Can you work these out from the model? Positions are in its coordinate system, mm. A direction names the side the tool comes from. Round coordinates to 2 decimals unless told otherwise and drop trailing zeros. Loops run counter-clockwise (first coordinate to the right, second up) from the corner with the lowest first, then second, coordinate; pieces in that order, holes last. Notation, with made-up numbers: M 14,8 L 44,8 A29 cw 44,47 Z; hole C 32.25,-32.5 d7. An arc over 180 degrees is marked long. Answer as CSV lines item,"result".
from build123d import *

# Parameters (mm, degrees)
SKETCH1_W           = 55.54
SKETCH1_H           = 50
SKETCH1_W_2         = 2
SKETCH1_H_2         = 16
SKETCH1_H_3         = 7
BOSS_EXTRUDE1_DEPTH = 2
SKETCH3_W           = 5
SKETCH3_H           = 2
CUT_EXTRUDE1_DEPTH  = 2
SKETCH4_W           = 6
SKETCH4_H           = 10
CUT_EXTRUDE2_DEPTH  = 2
CUT_EXTRUDE3_DEPTH  = 2


with BuildPart() as part:
    # Sketch1 → Boss-Extrude1 (new body)
    # profile 1 of 7: a face of its own
    with BuildSketch(Plane(origin=(0, 0, 0), x_dir=(1, 0, 0), z_dir=(0, 1, 0))):
        Rectangle(SKETCH1_W, SKETCH1_H)
        with Locations((18.77, 0)):
            Rectangle(SKETCH1_W_2, SKETCH1_H_2, mode=Mode.SUBTRACT)
    # profile 2 of 7: a face of its own
    with BuildSketch(Plane(origin=(0, 0, 0), x_dir=(1, 0, 0), z_dir=(0, 1, 0))):
        with Locations((28.77, 0)):
            Rectangle(SKETCH1_W_2, SKETCH1_H_3)
    # profile 3 of 7: a face of its own
    with BuildSketch(Plane(origin=(0, 0, 0), x_dir=(1, 0, 0), z_dir=(0, 1, 0))):
        with Locations((28.77, 15.5)):
            Rectangle(SKETCH1_W_2, SKETCH1_H_3)
    # profile 4 of 7: a face of its own
    with BuildSketch(Plane(origin=(0, 0, 0), x_dir=(1, 0, 0), z_dir=(0, 1, 0))):
        with Locations((28.77, -15.5)):
            Rectangle(SKETCH1_W_2, SKETCH1_H_3)
    # profile 5 of 7: a face of its own
    with BuildSketch(Plane(origin=(0, 0, 0), x_dir=(1, 0, 0), z_dir=(0, 1, 0))):
        with Locations((-28.77, 0)):
            Rectangle(SKETCH1_W_2, SKETCH1_H_3)
    # profile 6 of 7: a face of its own
    with BuildSketch(Plane(origin=(0, 0, 0), x_dir=(1, 0, 0), z_dir=(0, 1, 0))):
        with Locations((-28.77, -15.5)):
            Rectangle(SKETCH1_W_2, SKETCH1_H_3)
    # profile 7 of 7: a face of its own
    with BuildSketch(Plane(origin=(0, 0, 0), x_dir=(1, 0, 0), z_dir=(0, 1, 0))):
        with Locations((-28.77, 15.5)):
            Rectangle(SKETCH1_W_2, SKETCH1_H_3)
    extrude(amount=BOSS_EXTRUDE1_DEPTH)

    # Sketch3 → Cut-Extrude1 (cut)
    with BuildSketch(Plane(origin=(0, 2, 0), x_dir=(1, 0, 0), z_dir=(0, 1, 0))):
        with Locations((20.27, -22)):
            Rectangle(SKETCH3_W, SKETCH3_H)
        with Locations((20.27, 22)):
            Rectangle(SKETCH3_W, SKETCH3_H)
        with Locations((-20.27, 24)):
            Rectangle(SKETCH3_W, SKETCH3_H)
        with Locations((-20.27, -24)):
            Rectangle(SKETCH3_W, SKETCH3_H)
    extrude(amount=-CUT_EXTRUDE1_DEPTH, mode=Mode.SUBTRACT)

    # Sketch4 → Cut-Extrude2 (cut)
    with BuildSketch(Plane(origin=(0, 2, 0), x_dir=(1, 0, 0), z_dir=(0, 1, 0))):
        with Locations((-2.23, 0)):
            Rectangle(SKETCH4_W, SKETCH4_H)
    extrude(amount=-CUT_EXTRUDE2_DEPTH, mode=Mode.SUBTRACT)

    # Sketch5 → Cut-Extrude3 (cut)
    with BuildSketch(Plane(origin=(0, 2, 0), x_dir=(1, 0, 0), z_dir=(0, 1, 0))):
        Polygon((-19.496864222, 18.141064222), (-14.547116754, 13.191316754), (-15.961330317, 11.777103192), (-20.911077785, 16.72685066), align=None)
    extrude(amount=-CUT_EXTRUDE3_DEPTH, mode=Mode.SUBTRACT)


solid = part.part
Item 1: Will these pins go through, and if not, where does the flat tip stop? pin 1 (10 mm diameter, centred on x = -18, z = 15.5, fed in from -Y); pin 2 (1 mm diameter, centred on x = -29, y = 1, fed in from +Z); pin 3 (0.6 mm diameter, centred on x = -20, y = 1.5, fed in from +Z); pin 4 (0.6 mm diameter, centred on y = 1.5, z = 23.5, fed in from -X).
Output:
pin 1,"stops at y = 0"
pin 2,"stops at z = 19"
pin 3,"stops at z = 23"
pin 4,"stops at x = -27.77"
Item 2: On a 3-axis mill with a long thin cutter (end or side, diameter ignored), from which of +Z, -Z, +X, -X, +Y, -Y can I reach the whole of each face in a straight line? I mean faces 4 (the face through (5, 1, 25)), 5 (the face through (29, 1, -12)), 6 (the face through (-29, 1, 3.5)), 7 (the face through (-5.23, 1, 0)), 8 (the face through (-17.77, 1, 24)). Say none if no direction works.
Output:
face 4,"+Z, +X, -X, +Y, -Y"
face 5,"+X, +Y, -Y"
face 6,"-X, +Y, -Y"
face 7,"+Y, -Y"
face 8,"+Z, +Y, -Y"
Item 3: If we section it at D-D on z = -14.5: Write out the boundary of the cut face in (x, y).
Output:
outline,"M -29.77,0 L -18.68,0 L -18.68,2 L -29.77,2 Z; M -15.86,0 L 29.77,0 L 29.77,2 L -15.86,2 Z"
Item 4: We'd pull the mould along X, two halves only. Please class faces 1 (the face through (29.77, 1, 16)), 2 (the face through (-20, 1, -23)), 3 (the face through (-29, 1, -3.5)): released by +X, released by -X, zero draft, split by the parting line, or undercut.
Output:
face 1,"released by +X"
face 2,"undercut"
face 3,"zero draft"
Item 5: If we section it at A-A on z = -2: Write out the boundary of the cut face in (x, y), then the cut area to 3 significant figures.
Output:
outline,"M -29.77,0 L -5.23,0 L -5.23,2 L -29.77,2 Z; M 0.77,0 L 17.77,0 L 17.77,2 L 0.77,2 Z; M 19.77,0 L 29.77,0 L 29.77,2 L 19.77,2 Z"
area,"103 mm2"
Item 6: If I drill on line 1 along X through (y, z) = (0.6, 0); line 2 along Z through (x, y) = (22, 0.8); line 3 along X through (y, z) = (0.5, 21.5), over which ranges is the centre line in solid material (lowest first)? Write a range as from..to.
Output:
line 1,"x = -29.77..-5.23, 0.77..17.77, 19.77..29.77"
line 2,"z = -25..-23, -21..21, 23..25"
line 3,"x = -27.77..17.77, 22.77..27.77"
Item 7: If we section it at B-B on x = -3.5: Write out the boundary of the cut face in (y, z), then the cut area to 3 significant figures.
Output:
outline,"M 0,-25 L 2,-25 L 2,-5 L 0,-5 Z; M 0,5 L 2,5 L 2,25 L 0,25 Z"
area,"80.0 mm2"
Item 8: If we section it at C-C on x = 18.5: Write out the boundary of the cut face in (y, z).
Output:
outline,"M 0,-25 L 2,-25 L 2,-23 L 0,-23 Z; M 0,-21 L 2,-21 L 2,-8 L 0,-8 Z; M 0,8 L 2,8 L 2,21 L 0,21 Z; M 0,23 L 2,23 L 2,25 L 0,25 Z"
